```python
from build123d import *

# Parameters (mm, degrees)
F1_DEPTH = 2
F2_R     = 2.5
F3_DEPTH = 2.001


with BuildPart() as f1:
    # F0 (on Top) → F1 (new body)
    with BuildSketch(Plane.XY):
        with BuildLine():
            ThreePointArc((-1.5, 4.769696), (-2.95804, -4.031129), (5, 0))
            ThreePointArc((5, 0), (4.031129, 2.95804), (1.5, 4.769696))
            Line((1.5, 4.769696), (1.5, 0))
            Line((1.5, 0), (-1.5, 0))
            Line((-1.5, 0), (-1.5, 4.769696))
        make_face()
        with BuildLine():
            Line((1.5, 0), (1.5, 4.769696))
            ThreePointArc((1.5, 4.769696), (0, 5), (-1.5, 4.769696))
            Line((-1.5, 4.769696), (-1.5, 0))
            Line((-1.5, 0), (1.5, 0))
        make_face()
        with BuildLine():
            ThreePointArc((-1.5, 4.769696), (0, 5), (1.5, 4.769696))
            Line((1.5, 4.769696), (1.5, 73))
            Line((1.5, 73), (-1.5, 73))
            Line((-1.5, 73), (-1.5, 4.769696))
        make_face()
    extrude(amount=F1_DEPTH)

    # F2 (on face) → F3 (cut, through all)
    with BuildSketch(Plane.XY.offset(2)):
        Circle(F2_R)
    extrude(amount=-F3_DEPTH, mode=Mode.SUBTRACT)


solid = f1.part
```
Model file for the job. Use its own axes, mm. A direction names the side the tool comes from. Give positions to 0.01 mm unless a question says otherwise; leave off trailing zeros. Loops run counter-clockwise (first coordinate to the right, second up) from the corner with the lowest first, then second, coordinate; pieces in that order, holes last. Notation, with made-up numbers: (74.25, 2.25) -> (129.25, 2.25) arc R6 ccw to (129.25, 9.25) -> close; hole circle Ø8 at (-28, -16). An arc over 180 degrees is marked (long way). Use CSV: the item, a comma, the result in double quotes. Start each with the question number.
1) Slice it at C-C on y = 31.5. Give the cut face in (x, z), plus the area to 3 significant figures.
2) Slice it at D-D on x = -3.25. Give the cut face in (y, z), plus the area to 3 significant figures.
3) Wall check: line 1 (Y direction, x = 0, z = 0.7); line 2 (X direction, y = 53, z = 1.65); line 3 (Y direction, x = 2, z = 0.3). Give the ranges that are in metal, low to high.
4) Slice it at A-A on x = 0. Give the cut face in (y, z).
5) Flat gauge pins, fed straight in: pin 1 Ø6 at (x, y) = (0, 0) entering from -Z; pin 2 Ø0.6 at (y, z) = (51, 1) entering from +X. Where does each tip first touch, or does it go through?
6) Tool access for faces 1 (the flat face through (1, 31, 0)), 2 (the flat face through (-1.5, 39, 1)), 3 (the flat face through (1.5, 38, 1)): list every direction of +Z, -Z, +X, -X, +Y, -Y with a clear straight run to the whole face (end or side of a thin tool).
7) Slice it at B-B on z = 1.2. Give the cut face in (x, y), plus the area to 3 significant figures.
Computed values:
1,outline,"(-1.5, 0) -> (1.5, 0) -> (1.5, 2) -> (-1.5, 2) -> close"
1,area,"6.00 mm^2"
2,outline,"(-3.8, 0) -> (3.8, 0) -> (3.8, 2) -> (-3.8, 2) -> close"
2,area,"15.2 mm^2"
3,line 1,"y = -5 to -2.5, 2.5 to 73"
3,line 2,"x = -1.5 to 1.5"
3,line 3,"y = -4.58 to -1.5, 1.5 to 4.58"
4,outline,"(-5, 0) -> (-2.5, 0) -> (-2.5, 2) -> (-5, 2) -> close; (2.5, 0) -> (73, 0) -> (73, 2) -> (2.5, 2) -> close"
5,pin 1,"stops at z = 0"
5,pin 2,"stops at x = 1.5"
6,face 1,"-Z, +X, -X, +Y, -Y"
6,face 2,"+Z, -Z, -X, +Y"
6,face 3,"+Z, -Z, +X, +Y"
7,outline,"(-1.5, 4.77) arc R5 ccw (long way) to (1.5, 4.77) -> (1.5, 73) -> (-1.5, 73) -> close; hole circle Ø5 at (0, 0)"
7,area,"263 mm^2"
